Read the model definition and answer for the solid it produces. Units are mm, in the model's axes. Face numbers are marked on the shaded views. A direction names the side the tool comes from. Round coordinates to 2 decimals unless told otherwise and drop trailing zeros. Loops run counter-clockwise (first coordinate to the right, second up) from the corner with the lowest first, then second, coordinate; pieces in that order, holes last. Notation, with made-up numbers: (44.25, 54) - (57.25, 54) arc R18 cw to (57.25, 67) - close; hole circle Ø3 at (84, 80.25). An arc over 180 degrees is marked (long way). Use CSV: the item, a comma, the result in double quotes. Start each with the question number.
1. Given pin 1 Ø3.5 at (x, y) = (0, -18.796) entering from +Z (3 decimals); pin 2 Ø3 at (x, y) = (0.5, -11) entering from -Z; pin 3 Ø3 at (x, y) = (8, -7) entering from +Z; pin 4 Ø8 at (y, z) = (-2, 0.5) entering from -X, each flat-ended and moving along its own axis, determine where each tip first touches the part or whether it passes through.
2. Find section B-B (z = 5). Give the vertices of the cut face in (x, y).
3. Consider line 1 along Z through (x, y) = (0, 2.5); line 2 along Z through (x, y) = (1, -18) (3 decimals); line 3 along Y through (x, z) = (5, -4). Determine where each line is inside the solid, lowest interval first.
4. Find section D-D (z = -23.5). Give the vertices of the cut face in (x, y).
5. A tool of negligible diameter and unlimited length cuts with its end or side. For the marked faces 1, 2, 3 and 4, from which of +Z, -Z, +X, -X, +Y, -Y can it reach the whole face along a straight path? Write none if from no direction.
6. Find section A-A (x = 15). Give the vertices of the cut face in (y, z) (3 decimals), and give its area (3 significant figures).
from build123d import *

# Parameters (mm, degrees)
SKETCH2_W           = 11.938
SKETCH2_H           = 3.937
SKETCH2_W_2         = 9.652
SKETCH2_H_2         = 1.5875
SKETCH3_R           = 1.0795
BOSS_EXTRUDE2_DEPTH = 0.635
CIRPATTERN1_COUNT   = 4


with BuildPart() as part:
    # Sketch2 → Revolve1 (revolve)
    with BuildSketch(Plane(origin=(0, 0, 0), x_dir=(0, 0, -1), z_dir=(1, 0, 0)), mode=Mode.PRIVATE) as revolve1_sk:
        Polygon((-16.1925, 0), (16.1925, 0), (16.1925, 3.937), (16.1925, 8.128), (12.7, 13.97), (-12.7, 13.97), (-16.1925, 8.128), (-16.1925, 3.4925), (-17.5895, 3.4925), (-17.5895, 0), align=None)
        with Locations((22.1615, 1.9685)):
            Rectangle(SKETCH2_W, SKETCH2_H)
        with Locations((32.9565, 0.79375)):
            Rectangle(SKETCH2_W_2, SKETCH2_H_2)
    revolve(revolve1_sk.sketch.rotate(Axis((0, 0, 16.1925), (0, 0, -1)), 180), axis=Axis((0, 0, 16.1925), (0, 0, -1)))

    # Sketch3 → Boss-Extrude2 (add, symmetric)
    with BuildSketch(Plane.XY):
        with BuildLine():
            Line((-3.556, 17.065839525), (-3.556, 13.509839525))
            ThreePointArc((-3.556, 13.509839525), (0, 13.97), (3.556, 13.509839525))
            Line((3.556, 13.509839525), (3.556, 17.065839525))
            ThreePointArc((3.556, 17.065839525), (2.514471721, 19.580311232), (2.1e-08, 20.621839525))
            ThreePointArc((2.1e-08, 20.621839525), (-2.514471707, 19.580311247), (-3.556, 17.065839525))
        make_face()
        with Locations((0, 18.796)):
            Circle(SKETCH3_R, mode=Mode.SUBTRACT)
    boss_extrude2 = extrude(amount=BOSS_EXTRUDE2_DEPTH, both=True)

    # CirPattern1: Boss-Extrude2 ×4 about axis
    cirpattern1_axis = Axis((0, 0, 0), (0, 0, 1))
    for i in range(1, CIRPATTERN1_COUNT):
        add(boss_extrude2.rotate(cirpattern1_axis, i * 360 / CIRPATTERN1_COUNT))


solid = part.part
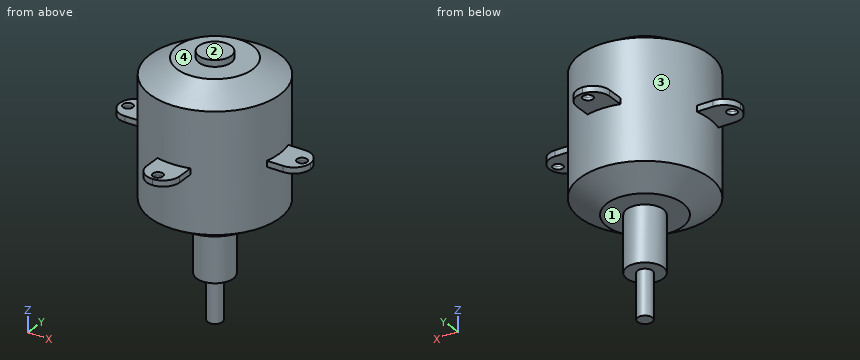
Filled sheet:
1,pin 1,"stops at z = 0.635"
1,pin 2,"stops at z = -15.37"
1,pin 3,"stops at z = 15.59"
1,pin 4,"stops at x = -20.62"
2,outline,"circle Ø27.94 at (0, 0)"
3,line 1,"z = -28.13 to 17.59"
3,line 2,"z = -0.635 to 0.635"
3,line 3,"y = -13.04 to 13.04"
4,outline,"circle Ø7.87 at (0, 0)"
5,face 1,"-Z"
5,face 2,"+Z, +X, -X, +Y, -Y"
5,face 3,"none"
5,face 4,"+Z"
6,outline,"(-3.556, -0.635) - (3.556, -0.635) - (3.556, 0.635) - (-3.556, 0.635) - close"
6,area,"9.03 mm²"
